```python
from build123d import *

# Parameters (mm, degrees)
SKETCH2_W               = 390
SKETCH2_H               = 80
BOSS_EXTRUDE1_DEPTH     = 60
SKETCH4_W               = 350
SKETCH4_H               = 75
CUT_EXTRUDE1_DEPTH      = 40
SKETCH5_R               = 6
CUT_EXTRUDE2_DEPTH      = 360
CUT_EXTRUDE2_DEPTH_BACK = 10


with BuildPart() as part:
    # Sketch2 → Boss-Extrude1 (new body)
    with BuildSketch(Plane.XY):
        with Locations((195, 40)):
            Rectangle(SKETCH2_W, SKETCH2_H)
    extrude(amount=BOSS_EXTRUDE1_DEPTH)

    # Sketch4 → Cut-Extrude1 (cut)
    with BuildSketch(Plane.XY.offset(60)):
        with Locations((195, 42.5)):
            Rectangle(SKETCH4_W, SKETCH4_H)
    extrude(amount=-CUT_EXTRUDE1_DEPTH, mode=Mode.SUBTRACT)

    # Sketch5 → Cut-Extrude2 (cut, two sides)
    with BuildSketch(Plane(origin=(20, 0, 0), x_dir=(0, 0, -1), z_dir=(1, 0, 0))) as cut_extrude2_sk:
        with Locations((-38.957689145, 40)):
            Circle(SKETCH5_R)
    extrude(amount=CUT_EXTRUDE2_DEPTH, mode=Mode.SUBTRACT)
    extrude(cut_extrude2_sk.sketch, amount=-CUT_EXTRUDE2_DEPTH_BACK, mode=Mode.SUBTRACT)


solid = part.part
```
Verification items for the finished model (mm, model axes). A direction names the side the tool comes from. Coordinates: 2 decimals unless noted, no trailing zeros. Write each loop counter-clockwise with the first axis right and the second up, starting at its lowest first coordinate (ties: lowest second). Pieces come first, ordered by that corner, then holes. Notation, with made-up numbers: (89.25, -9) - (143.25, -9) arc R19 cw to (143.25, 27) - close; hole circle Ø1 at (48.25, 6). An arc over 180 degrees is marked (long way). One line per question, with ' | ' between items. Start each with the question number.
1. Material ranges on line 1 along X through (y, z) = (25, 45); line 2 along Y through (x, z) = (246, 25); line 3 along Z through (x, y) = (50.5, 69), recorded low to high.
2. Section check B-B (x = 187). Enter the section's corners in (y, z), plus the area to 3 significant figures.
3. Section check C-C (y = 73). Enter the section's corners in (x, z).
4. Section check A-A (y = 40). Enter the section's corners in (x, z).
5. Access from +Z, -Z, +X, -X, +Y, -Y to the whole of each face (thin tool, end or side, straight path). Record for faces 5 (the cylindrical face through (15.07, 40.264, 44.952)), 6 (the flat face through (194.1, 4.6, 60)), 7 (the flat face through (193, 43, 20)).
6. Gauge pin test, flat ends, axial feed: P1, Ø1.5, axis at x = 233.5, z = 42.5, coming from the +Y side; P2, Ø10, axis at x = 39.5, y = 56.5, coming from the +Z side. Record the tip position at first contact, or that the pin passes through.
7. Draft check along Y on faces 1 (the flat face through (380, 40, 39)), 2 (the flat face through (149, 80, 16)), 3 (the flat face through (370, 42, 45)), 4 (the cylindrical face through (374.93, 40.264, 44.952)). Enter one of: released by +Y, released by -Y, zero draft, split by the parting line, or undercut.
Computed values:
1) line 1: 0 to 20, 370 to 390 | line 2: 0 to 5 | line 3: 0 to 20
2) outline: (0, 0) - (80, 0) - (80, 20) - (5, 20) - (5, 60) - (0, 60) - close | area: 1,800 mm²
3) outline: (0, 0) - (390, 0) - (390, 60) - (370, 60) - (370, 20) - (20, 20) - (20, 60) - (0, 60) - close
4) outline: (0, 0) - (390, 0) - (390, 60) - (370, 60) - (370, 44.96) - (380, 44.96) - (380, 32.96) - (370, 32.96) - (370, 20) - (20, 20) - (20, 32.96) - (10, 32.96) - (10, 44.96) - (20, 44.96) - (20, 60) - (0, 60) - close
5) face 5: none | face 6: +Z, +X, -X, +Y, -Y | face 7: +Z, +Y
6) P1: y = 5 | P2: z = 20
7) face 1: undercut | face 2: released by +Y | face 3: zero draft | face 4: undercut
